Drawing for the job (mm, zero at the part's lowest x, y, z). Round coordinates to 2 decimals unless told otherwise and drop trailing zeros. Write each loop counter-clockwise with the first axis right and the second up, starting at its lowest first coordinate (ties: lowest second). Pieces come first, ordered by that corner, then holes. Notation, with made-up numbers: M -12.75,1.25 L 18.25,1.25 A30 cw 18.25,27.25 Z; hole C 81,87 d6. An arc over 180 degrees is marked long. Use a Markdown table: item, result.
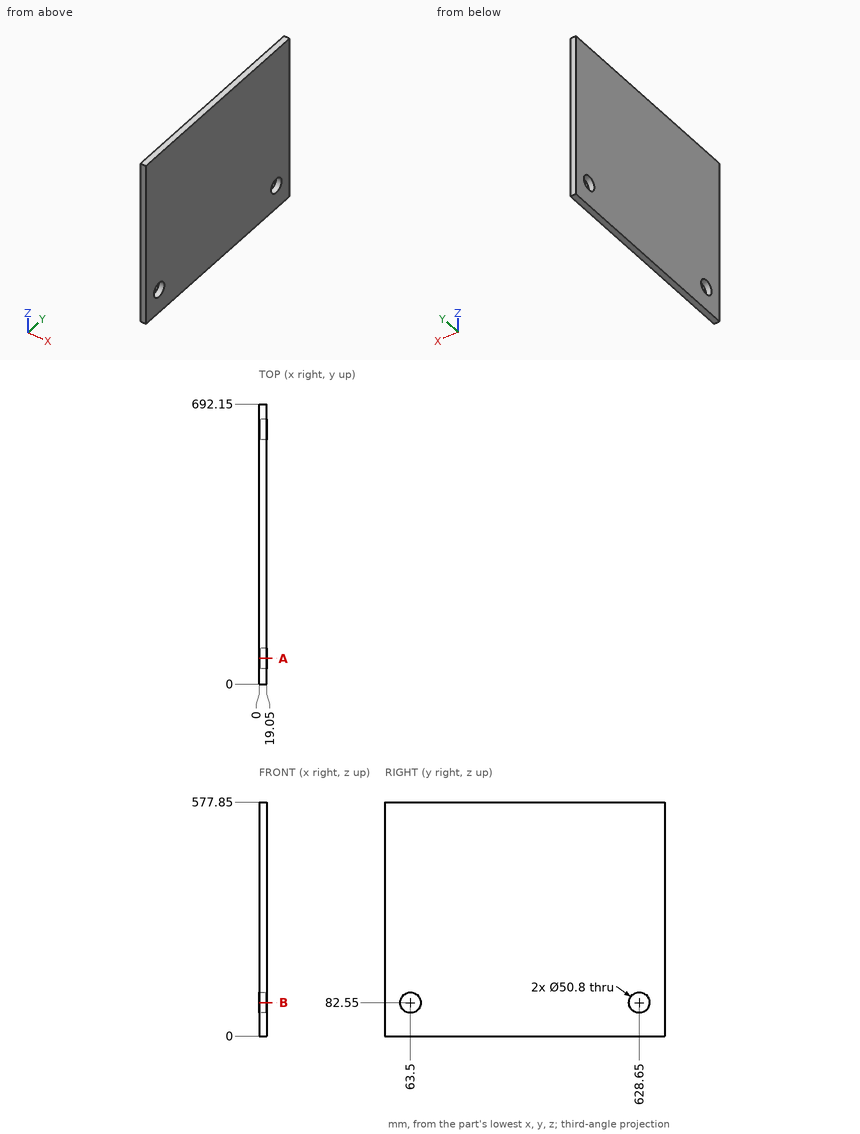
Q1. Drop a flat-ended pin along its axis: P1, Ø2, axis at x = 8.5, y = 490.5, coming from the -Z side. Give the stop position or say it passes through.
Response values:
| item | result |
|---|---|
| P1 | stops at z = 0 |
Q2. Cut at B-B on z = 82.55. Give the cut face in (x, y).
Response values:
| item | result |
|---|---|
| outline | M 0,0 L 19.05,0 L 19.05,38.1 L 0,38.1 Z; M 0,88.9 L 19.05,88.9 L 19.05,603.25 L 0,603.25 Z; M 0,654.05 L 19.05,654.05 L 19.05,692.15 L 0,692.15 Z |
Q3. Cut at A-A on y = 63.5. Give the cut face in (x, z), and give its area (3 significant figures).
Response values:
| item | result |
|---|---|
| outline | M 0,0 L 19.05,0 L 19.05,57.15 L 0,57.15 Z; M 0,107.95 L 19.05,107.95 L 19.05,577.85 L 0,577.85 Z |
| area | 10,000 mm2 |
Q4. Drill centre lines: L1, parallel to Y at x = 13.25, z = 82.55; L2, parallel to Y at x = 8, z = 67. Where is each one in solid material? Low to high.
Response values:
| item | result |
|---|---|
| L1 | y = 0 to 38.1, 88.9 to 603.25, 654.05 to 692.15 |
| L2 | y = 0 to 43.42, 83.58 to 608.57, 648.73 to 692.15 |
